from build123d import *

# Parameters (mm, degrees)
PAD_DEPTH       = 1
SKETCH002_W     = 71.8
SKETCH002_H     = 45
PAD001_DEPTH    = 3
SKETCH003_W     = 6.9
SKETCH003_H     = 22.7
SKETCH003_W_2   = 5.08
SKETCH003_H_2   = 38.099998
SKETCH003_W_3   = 15.24
SKETCH003_H_3   = 2.54
POCKET_DEPTH    = 1.2
SKETCH004_W     = 1.2
SKETCH004_H     = 6.35
PAD002_DEPTH    = 3.3
SKETCH008_W     = 5
SKETCH008_H     = 2.3
POCKET001_DEPTH = 0.5
SKETCH009_W     = 5
SKETCH009_H     = 2.3
POCKET002_DEPTH = 0.5
CHAMFER002_SIZE = 2


with BuildPart() as part:
    # Sketch001 → Pad (new body)
    with BuildSketch(Plane.XY):
        Polygon((-66.6, 20.1), (-66.6, -20.1), (-2.9, -20.1), (-2.9, -11.35), (4, -11.35), (4, -22.5), (-67.8, -22.5), (-67.8, 22.5), (4, 22.5), (4, 11.35), (-2.9, 11.35), (-2.9, 20.1), align=None)
    extrude(amount=PAD_DEPTH)

    # Sketch002 (on Face13 of Pad) → Pad001 (join)
    with BuildSketch(Plane(origin=(0, 0, 0), x_dir=(1, 0, 0), z_dir=(0, 0, -1))):
        with Locations((-31.9, 0)):
            Rectangle(SKETCH002_W, SKETCH002_H)
    extrude(amount=PAD001_DEPTH)

    # Sketch003 (on Face4 of Pad001) → Pocket (cut)
    with BuildSketch(Plane.XY):
        with Locations((0.55, 0)):
            Rectangle(SKETCH003_W, SKETCH003_H)
        with Locations((-12, 0)):
            Rectangle(SKETCH003_W_2, SKETCH003_H_2)
        with Locations((-55, 18)):
            Rectangle(SKETCH003_W_3, SKETCH003_H_3)
        with Locations((-55.5, -18)):
            Rectangle(SKETCH003_W_3, SKETCH003_H_3)
        with Locations((-37, -18)):
            Rectangle(SKETCH003_W_3, SKETCH003_H_3)
    extrude(amount=-POCKET_DEPTH, mode=Mode.SUBTRACT)

    # Sketch004 (on Face5 of Pocket) → Pad002 (join)
    with BuildSketch(Plane.XY.offset(1)):
        with Locations((-67.2, -0.625)):
            Rectangle(SKETCH004_W, SKETCH004_H)
        Polygon((-67.8, 11.95), (-66.6, 11.95), (-66.6, 20.1), (-2.9, 20.1), (-2.9, 11.35), (4, 11.35), (4, 21.1), (-67.8, 21.1), align=None)
        Polygon((-67.8, -13.2), (-66.6, -13.2), (-66.6, -20.1), (-2.9, -20.1), (-2.9, -11.35), (4, -11.35), (4, -21.1), (-67.8, -21.1), align=None)
    extrude(amount=PAD002_DEPTH)

    # Sketch008 (on Face12 of Pad002) → Pocket001 (cut)
    with BuildSketch(Plane(origin=(0, 21.1, 0), x_dir=(-1, 0, 0), z_dir=(0, 1, 0))):
        with Locations((63.8, 2.65)):
            Rectangle(SKETCH008_W, SKETCH008_H)
        with Locations((0, 2.65)):
            Rectangle(SKETCH008_W, SKETCH008_H)
    extrude(amount=-POCKET001_DEPTH, mode=Mode.SUBTRACT)

    # Sketch009 (on Face2 of Pocket001) → Pocket002 (cut)
    with BuildSketch(Plane.XZ.offset(21.1)):
        with Locations((-63.8, 2.65)):
            Rectangle(SKETCH009_W, SKETCH009_H)
        with Locations((0, 2.65)):
            Rectangle(SKETCH009_W, SKETCH009_H)
    extrude(amount=-POCKET002_DEPTH, mode=Mode.SUBTRACT)

    # Chamfer002
    chamfer002_edges = [part.edges().sort_by_distance(p)[0] for p in [
        (-31.9, 22.5, -3),
        (-31.9, -22.5, -3),
    ]]
    chamfer(chamfer002_edges, length=CHAMFER002_SIZE)


solid = part.part
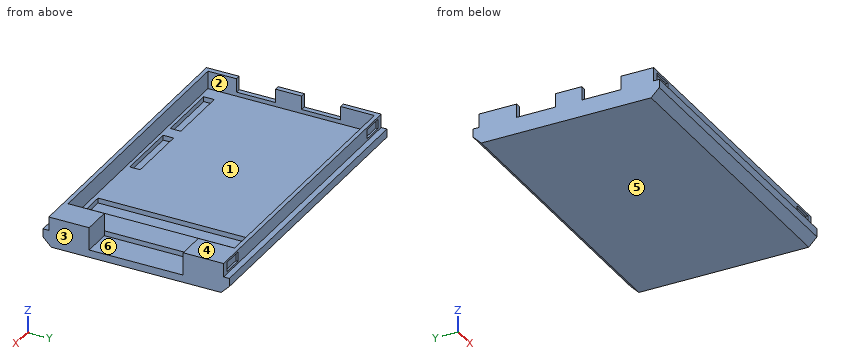
Can you work these out from the model? Positions are in its coordinate system, mm. Face numbers are marked on the shaded views. A direction names the side the tool comes from. Give positions to 0.01 mm unless a question says otherwise; leave off trailing zeros. Loops run counter-clockwise (first coordinate to the right, second up) from the corner with the lowest first, then second, coordinate; pieces in that order, holes last. Notation, with made-up numbers: M -37,28.5 L 19,28.5 A25 ccw 19,53.5 Z; hole C 14,71.25 d10. An arc over 180 degrees is marked long. One line per item, written item: value. Start each with the question number.
1) On a 3-axis mill with a long thin cutter (end or side, diameter ignored), from which of +Z, -Z, +X, -X, +Y, -Y can I reach the whole of each face in a straight line? I mean the marked faces 5 and 6. Say none if no direction works.
2) If I drill on line 1 (X direction, y = 14.5, z = 1); line 2 (Y direction, x = -58.5, z = 2); line 3 (X direction, y = -2.5, z = -0.5), over which ranges is the centre line in solid material (lowest first)? Write a range as [from, to].
3) If we section it at D-D, the plane z = -2.25: Write out the boundary of the cut face in (x, y), and give its area (3 significant figures).
4) If we section it at C-C, the plane z = 2.5: Give the number of separate pieces and of enclosed holes in the cut face, and give its area (3 significant figures).
5) If we section it at B-B, the plane y = -6: Write out the boundary of the cut face in (x, z).
6) I'm going to push flat-ended pins straight in: pin 1 (1 mm diameter, centred on x = -67.5, z = 2, fed in from +Y); pin 2 (2 mm diameter, centred on y = -5.5, z = 1.5, fed in from +X); pin 3 (1.3 mm diameter, centred on x = -34, y = -18.5, fed in from +Z). Where does each tip first touch, or does it pass through?
7) If we section it at A-A, the plane x = -11.5: Write out the boundary of the cut face in (y, z), and give its area (3 significant figures).
8) Thinking about a two-plate mould opening in X: for the marked faces 1, 2, 3 and 4, which applies, +X half, -X half, draft (parallel to the pull), parting line (faces both ways), or undercut?
Completed:
1. face 5: -Z, +X, -X, +Y, -Y
1. face 6: +Z, +X
2. line 1: x = [-67.8, -66.6], [-2.9, 4]
2. line 2: y = [-21.1, -20.1], [20.1, 21.1]
2. line 3: x = [-67.8, -14.54], [-9.46, -2.9]
3. outline: M -67.8,-21.25 L 4,-21.25 L 4,21.25 L -67.8,21.25 Z
3. area: 3,050 mm^2
4. separate pieces: 3
4. enclosed holes: 0
4. area: 280 mm^2
5. outline: M -67.8,-3 L 4,-3 L 4,-1.2 L -2.9,-1.2 L -2.9,0 L -9.46,0 L -9.46,-1.2 L -14.54,-1.2 L -14.54,0 L -66.6,0 L -66.6,1 L -67.8,1 Z
6. pin 1: stops at y = 21.1
6. pin 2: stops at x = -66.6
6. pin 3: stops at z = -1.2
7. outline: M -22.5,-1 L -20.5,-3 L 20.5,-3 L 22.5,-1 L 22.5,1 L 21.1,1 L 21.1,4.3 L 20.1,4.3 L 20.1,0 L 19.05,0 L 19.05,-1.2 L -19.05,-1.2 L -19.05,0 L -20.1,0 L -20.1,4.3 L -21.1,4.3 L -21.1,1 L -22.5,1 Z
7. area: 96.7 mm^2
8. face 1: undercut
8. face 2: undercut
8. face 3: +X half
8. face 4: draft
